Can you work these out from the drawing? Everything is in mm from the part's minimum corner. A direction names the side the tool comes from. Round coordinates to 2 decimals unless told otherwise and drop trailing zeros. Loops run counter-clockwise (first coordinate to the right, second up) from the corner with the lowest first, then second, coordinate; pieces in that order, holes last. Notation, with made-up numbers: (74, -8.75) - (88, -8.75) arc R13 ccw to (88, -1.75) - close; hole circle Ø5 at (0, -14). An arc over 180 degrees is marked (long way). Put each result on its own line as item: value. Start each with the question number.
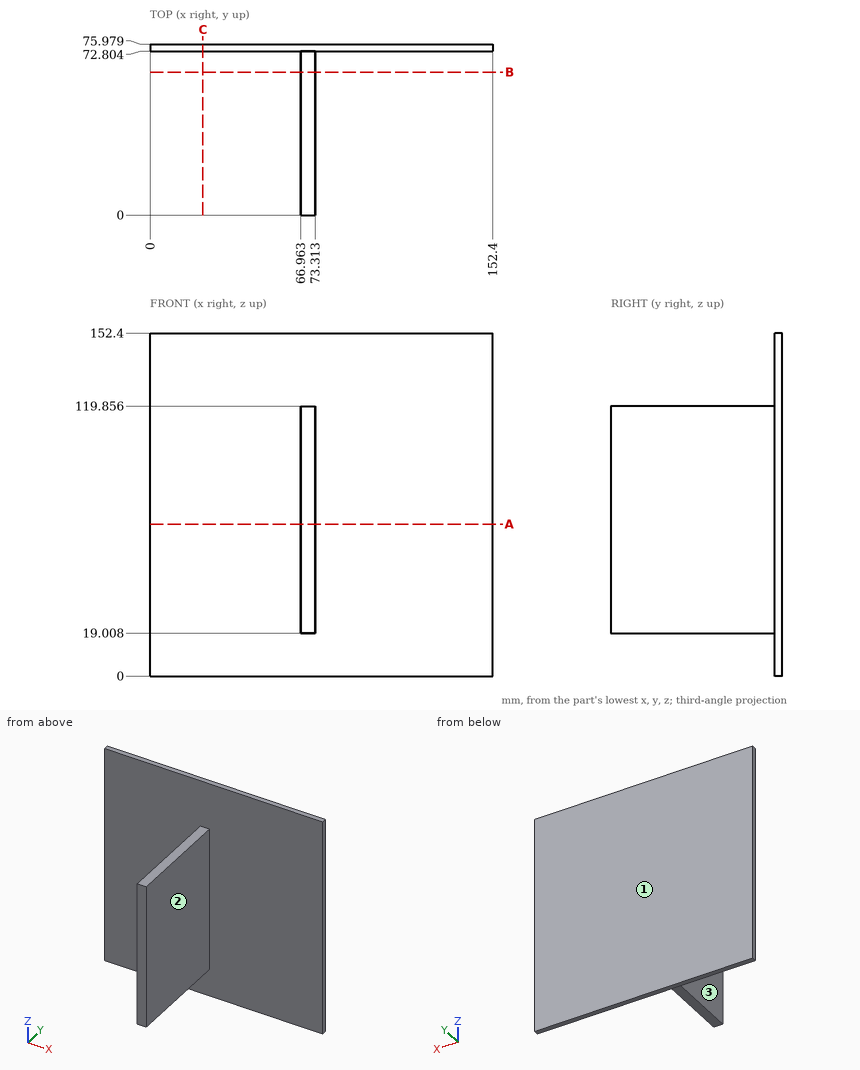
Item 1: Suppose I cut it at B-B, the plane y = 63.5. List the corners of the cut face in (x, z) for me.
Item 2: Suppose I cut it at C-C, the plane x = 23.5. List the corners of the cut face in (y, z) for me, then the cut area to 3 significant figures.
Item 3: Will these pins go through, and if not, where does the flat tip stop? P1, Ø5, axis at x = 71, y = 19.5, coming from the -Z side; P2, Ø1.5, axis at y = 66, z = 35.5, coming from the -X side; P3, Ø22, axis at y = 45.5, z = 87.5, coming from the +X side.
Item 4: Suppose I cut it at A-A, the plane z = 67.5. List the corners of the cut face in (x, y) for me.
Item 5: On a 3-axis mill with a long thin cutter (end or side, diameter ignored), from which of +Z, -Z, +X, -X, +Y, -Y can I reach the whole of each face in a straight line? I mean the marked faces 1, 2 and 3. Say none if no direction works.
Item 6: I need wall thicknesses on line 1 (Y direction, x = 14.5, z = 22); line 2 (X direction, y = 67, z = 46). Which ranges of each line are inside material? Lowest first, please. Write a range as from..to.
Numbers:
1. outline: (66.96, 19.01) - (73.31, 19.01) - (73.31, 119.86) - (66.96, 119.86) - close
2. outline: (72.8, 0) - (75.98, 0) - (75.98, 152.4) - (72.8, 152.4) - close
2. area: 484 mm^2
3. P1: z = 19.01
3. P2: x = 66.96
3. P3: x = 73.31
4. outline: (0, 72.8) - (66.96, 72.8) - (66.96, 0) - (73.31, 0) - (73.31, 72.8) - (152.4, 72.8) - (152.4, 75.98) - (0, 75.98) - close
5. face 1: +Z, -Z, +X, -X, +Y
5. face 2: +Z, -Z, +X, -Y
5. face 3: +Z, -Z, -X, -Y
6. line 1: 72.8..75.98
6. line 2: 66.96..73.31
